from build123d import *

# Parameters (mm, degrees)
MAIN_DEPTH                = 11.25
SKETCH2_R                 = 1.25
FIXHOLE1_DEPTH            = 83
SKETCH3_R                 = 1.25
FIXHOLE2_DEPTH            = 83
SKETCH6_R                 = 1.25
CUT_EXTRUDE2_DEPTH        = 63.932503526
LPATTERN1_COUNT           = 5
LPATTERN1_PITCH           = 20
SKETCH7_R                 = 5
BOSS_EXTRUDE1_DEPTH       = 3
SKETCH8_R                 = 1.25
CUT_EXTRUDE3_DEPTH        = 66.932503526
LPATTERN2_COUNT           = 2
LPATTERN2_PITCH           = 12.5
LPATTERN2_COPY_1_SKETCH_R = 1.25
LPATTERN2_COPY_1_DEPTH    = 63.932503526
LPATTERN2_COPY_2_SKETCH_R = 1.25
LPATTERN2_COPY_2_DEPTH    = 63.932503526
LPATTERN2_COPY_3_SKETCH_R = 1.25
LPATTERN2_COPY_3_DEPTH    = 63.932503526
LPATTERN2_COPY_4_SKETCH_R = 1.25
LPATTERN2_COPY_4_DEPTH    = 63.932503526


with BuildPart() as part:
    # Sketch1 → Main (new body, symmetric)
    with BuildSketch(Plane.XY):
        Polygon((-41, -41), (41, 41), (41, 39), (51, 39), (51, 34), (41, 34), (-34, -41), (-34, -51), (-39, -51), (-39, -41), align=None)
    extrude(amount=MAIN_DEPTH, both=True)

    # Sketch2 → FixHole1 (cut, through all)
    with BuildSketch(Plane(origin=(41, 0, 0), x_dir=(0, 0, -1), z_dir=(1, 0, 0))):
        with Locations((0, -46)):
            Circle(SKETCH2_R)
    extrude(amount=-FIXHOLE1_DEPTH, mode=Mode.SUBTRACT)

    # Sketch3 → FixHole2 (cut, through all)
    with BuildSketch(Plane(origin=(0, -41, 0), x_dir=(-1, 0, 0), z_dir=(0, -1, 0))):
        with Locations((-46, 0)):
            Circle(SKETCH3_R)
    extrude(amount=-FIXHOLE2_DEPTH, mode=Mode.SUBTRACT)

    # Sketch6 → Cut-Extrude2 (cut, through all)
    with BuildSketch(Plane(origin=(3.5, -3.5, 0), x_dir=(0, 0, 1), z_dir=(-0.707106781, 0.707106781, 0))):
        with Locations((-6.25, 40)):
            Circle(SKETCH6_R)
    cut_extrude2 = extrude(amount=CUT_EXTRUDE2_DEPTH, mode=Mode.SUBTRACT)

    # LPattern1: Cut-Extrude2 ×5
    with Locations(*[Vector(-0.707106781, -0.707106781, 0) * (i * LPATTERN1_PITCH) for i in range(1, LPATTERN1_COUNT)]):
        add(cut_extrude2, mode=Mode.SUBTRACT)

    # Sketch7 → Boss-Extrude1 (add)
    with BuildSketch(Plane(origin=(3.5, -3.5, 0), x_dir=(0, 0, 1), z_dir=(-0.707106781, 0.707106781, 0))):
        with Locations((-6.25, -33.008531019)):
            Circle(SKETCH7_R)
        with Locations((-6.25, 31.791468981)):
            Circle(SKETCH7_R)
    boss_extrude1 = extrude(amount=-BOSS_EXTRUDE1_DEPTH)

    # Sketch8 → Cut-Extrude3 (cut, through all)
    with BuildSketch(Plane(origin=(5.621320344, -5.621320344, 0), x_dir=(0, 0, -1), z_dir=(0.707106781, -0.707106781, 0))):
        with Locations((6.25, 31.791468981)):
            Circle(SKETCH8_R)
        with Locations((6.25, -33.008531019)):
            Circle(SKETCH8_R)
    cut_extrude3 = extrude(amount=-CUT_EXTRUDE3_DEPTH, mode=Mode.SUBTRACT)

    # LPattern2: Boss-Extrude1, Cut-Extrude3, Cut-Extrude2 ×2
    with Locations(*[(0, 0, i * LPATTERN2_PITCH) for i in range(1, LPATTERN2_COUNT)]):
        add(boss_extrude1)
        add(cut_extrude3, mode=Mode.SUBTRACT)
        add(cut_extrude2, mode=Mode.SUBTRACT)

    # LPattern2 copy 1 sketch → LPattern2 copy 1 (cut, through all)
    with BuildSketch(Plane(origin=(-10.642135624, -17.642135624, 12.5), x_dir=(0, 0, 1), z_dir=(-0.707106781, 0.707106781, 0))):
        with Locations((-6.25, 40)):
            Circle(LPATTERN2_COPY_1_SKETCH_R)
    extrude(amount=LPATTERN2_COPY_1_DEPTH, mode=Mode.SUBTRACT)

    # LPattern2 copy 2 sketch → LPattern2 copy 2 (cut, through all)
    with BuildSketch(Plane(origin=(-24.784271247, -31.784271247, 12.5), x_dir=(0, 0, 1), z_dir=(-0.707106781, 0.707106781, 0))):
        with Locations((-6.25, 40)):
            Circle(LPATTERN2_COPY_2_SKETCH_R)
    extrude(amount=LPATTERN2_COPY_2_DEPTH, mode=Mode.SUBTRACT)

    # LPattern2 copy 3 sketch → LPattern2 copy 3 (cut, through all)
    with BuildSketch(Plane(origin=(-38.926406871, -45.926406871, 12.5), x_dir=(0, 0, 1), z_dir=(-0.707106781, 0.707106781, 0))):
        with Locations((-6.25, 40)):
            Circle(LPATTERN2_COPY_3_SKETCH_R)
    extrude(amount=LPATTERN2_COPY_3_DEPTH, mode=Mode.SUBTRACT)

    # LPattern2 copy 4 sketch → LPattern2 copy 4 (cut, through all)
    with BuildSketch(Plane(origin=(-53.068542495, -60.068542495, 12.5), x_dir=(0, 0, 1), z_dir=(-0.707106781, 0.707106781, 0))):
        with Locations((-6.25, 40)):
            Circle(LPATTERN2_COPY_4_SKETCH_R)
    extrude(amount=LPATTERN2_COPY_4_DEPTH, mode=Mode.SUBTRACT)


solid = part.part
Build history of the part. All positions in model axes, mm. A direction names the side the tool comes from. Coordinates: 2 decimals unless noted, no trailing zeros. Order: outer loops, then holes, each group sorted by start corner. A loop starts at its lowest first (then second) coordinate and runs counter-clockwise, first axis right, second up. Notation, with made-up numbers: (38.5, 83) - (72.5, 83) arc R25 ccw to (72.5, 103) - close; hole circle Ø4 at (-30.5, 37.5). An arc over 180 degrees is marked (long way). Write item = value, one per line. Start each with the question number.
1) Saw through at B-B on x = 46. Write the cut outline in (y, z), then the cut area to 3 significant figures.
2) Two-plate mould, pull along Z, no slides. Class faces 1 (the face through (47.25, 36.47, -0.05)), 2 (the face through (2, -1, -11.25)), 3 (the face through (-36, -51, 0)), 4 (the face through (2, -1, 11.25)): pulls with the +Z half, pulls with the -Z half, needs draft (parallel to the pull), parting line crosses it, or undercut.
3) Saw through at D-D on x = 9. Write the cut outline in (y, z).
4) Wall check: line 1 along Z through (x, y) = (46, 35.75); line 2 along Y through (x, z) = (44.5, -7.75); line 3 along Y through (x, z) = (-37.7, 0). Give the ranges that are in metal, low to high. Write a range as from..to.
5) 3-axis set-ups, long thin cutter, end or side, ignore diameter. For faces 5 (the face through (-34, -48, 0)), 6 (the face through (-40, -41, 0)), 7 (the face through (-19.893, -25.593, 7.171)): which of +Z, -Z, +X, -X, +Y, -Y reach the whole face in a straight line?
6) Flat gauge pins, fed straight in: pin 1 Ø4 at (x, z) = (17.5, -8.5) entering from -Y; pin 2 Ø5 at (x, z) = (44, 4.5) entering from +Y; pin 3 Ø4 at (y, z) = (-22, 6) entering from -X. Where does each tip first touch, or does it go through?
7) Saw through at A-A on y = -46. Write the cut outline in (x, z), then the cut area to 3 significant figures.
8) Saw through at C-C on z = -3.25. Write the cut outline in (x, y), then the cut area to 4 significant figures.
From the geometry:
q1.outline = (34, -11.25) - (39, -11.25) - (39, -1.25) - (34, -1.25) - close; (34, 1.25) - (39, 1.25) - (39, 11.25) - (34, 11.25) - close
q1.area = 100 mm^2
q2.face_1 = undercut
q2.face_2 = pulls with the -Z half
q2.face_3 = needs draft
q2.face_4 = pulls with the +Z half
q3.outline = (2, -11.25) - (9, -11.25) - (9, 11.25) - (2, 11.25) - close
q4.line_1 = -11.25..-1.25, 1.25..11.25
q4.line_2 = 34..39
q4.line_3 = -51..-47.25, -44.75..-37.7
q5.face_5 = +Z, -Z, +X, -Y
q5.face_6 = +Z, -Z, -X, -Y
q5.face_7 = none
q6.pin_1 = 8.5
q6.pin_2 = 39
q6.pin_3 = -23.84
q7.outline = (-39, -11.25) - (-34, -11.25) - (-34, -1.25) - (-39, -1.25) - close; (-39, 1.25) - (-34, 1.25) - (-34, 11.25) - (-39, 11.25) - close
q7.area = 100 mm^2
q8.outline = (-41, -41) - (-39, -41) - (-39, -51) - (-34, -51) - (-34, -41) - (-22.67, -29.67) - (-20.55, -31.79) - (-14.89, -26.13) - (-17.01, -24.01) - (23.15, 16.15) - (25.27, 14.03) - (30.93, 19.69) - (28.81, 21.81) - (41, 34) - (51, 34) - (51, 39) - (41, 39) - (41, 41) - close
q8.area = 697.5 mm^2
